```python
from build123d import *

# Parameters (mm, degrees)
F0_W     = 15
F0_H     = 15
F1_DEPTH = 5
F2_R     = 2.5
F3_DEPTH = 15
F4_R     = 2.5
F5_DEPTH = 15


with BuildPart() as f1:
    # F0 (on Front) → F1 (new body, symmetric)
    with BuildSketch(Plane.XZ):
        Rectangle(F0_W, F0_H)
    extrude(amount=F1_DEPTH, both=True)

    # F2 (on face) → F3 (cut, through all)
    with BuildSketch(Plane.YZ.offset(7.5)):
        Circle(F2_R)
    extrude(amount=-F3_DEPTH, mode=Mode.SUBTRACT)

    # F4 (on face) → F5 (cut, through all)
    with BuildSketch(Plane.XY.offset(7.5)):
        Circle(F4_R)
    extrude(amount=-F5_DEPTH, mode=Mode.SUBTRACT)


solid = f1.part
```
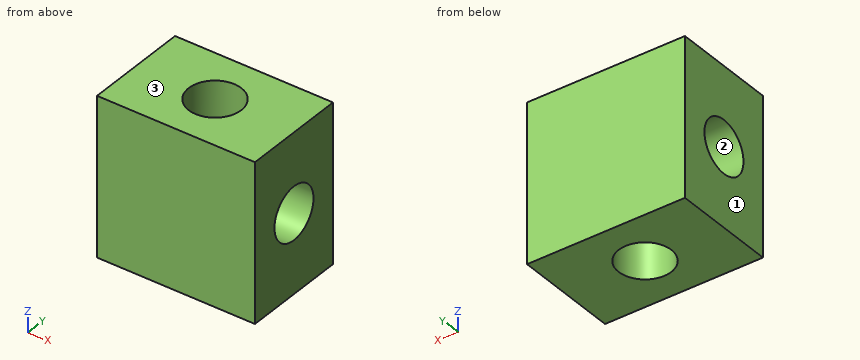
Design review of the part built by this model. Coordinates are the model's own, in mm. Face numbers are marked on the shaded views. Coordinates: 2 decimals unless noted, no trailing zeros. Order: outer loops, then holes, each group sorted by start corner. A loop starts at its lowest first (then second) coordinate and runs counter-clockwise, first axis right, second up.
1) Wall thickness on line 1 along X through (y, z) = (0, 5.5); line 2 along Z through (x, y) = (4.25, 0.5): over which ranges is each line inside the solid? List them lowest first.
2) Take a section at B-B, the plane z = -1. Give the boundary of the cut face in (x, y), and give its area (3 significant figures).
3) Mouldability with a two-part tool opening along Z and no side actions: class the marked faces 1, 2 and 3 as +Z half, -Z half, draft (parallel to the pull), parting line (faces both ways), or undercut.
4) Take a section at D-D, the plane z = 5. Give the boundary of the cut face in (x, y).
5) Take a section at C-C, the plane x = -3.5. Give the boundary of the cut face in (y, z), and give its area (3 significant figures).
6) Take a section at A-A, the plane y = 0. Give the boundary of the cut face in (x, z).
Returned:
1. line 1: x = -7.5 to -2.5, 2.5 to 7.5
1. line 2: z = -7.5 to -2.45, 2.45 to 7.5
2. outline: (-7.5, -5) - (7.5, -5) - (7.5, -2.29) - (1, -2.29) arc R2.5 cw to (-1, -2.29) - (-7.5, -2.29) - close; (-7.5, 2.29) - (-1, 2.29) arc R2.5 cw to (1, 2.29) - (7.5, 2.29) - (7.5, 5) - (-7.5, 5) - close
2. area: 80.7 mm2
3. face 1: draft
3. face 2: undercut
3. face 3: +Z half
4. outline: (-7.5, -5) - (7.5, -5) - (7.5, 5) - (-7.5, 5) - close; hole circle Ø5 at (0, 0)
5. outline: (-5, -7.5) - (5, -7.5) - (5, 7.5) - (-5, 7.5) - close; hole circle Ø5 at (0, 0)
5. area: 130 mm2
6. outline: (-7.5, -7.5) - (-2.5, -7.5) - (-2.5, -2.5) - (-7.5, -2.5) - close; (-7.5, 2.5) - (-2.5, 2.5) - (-2.5, 7.5) - (-7.5, 7.5) - close; (2.5, -7.5) - (7.5, -7.5) - (7.5, -2.5) - (2.5, -2.5) - close; (2.5, 2.5) - (7.5, 2.5) - (7.5, 7.5) - (2.5, 7.5) - close
